from build123d import *

# Parameters (mm, degrees)
SKETCH2_R           = 14
BOSS_EXTRUDE1_DEPTH = 24
SKETCH3_R           = 3.95
BOSS_EXTRUDE2_DEPTH = 7
SKETCH4_R           = 3
BOSS_EXTRUDE3_DEPTH = 7
SKETCH6_R           = 1.25
CUT_EXTRUDE1_DEPTH  = 5
EXTRUDE_START       = 3
SKETCH_1_R          = 3
EXTRUDE_1_DEPTH     = 3
CUT_EXTRUDE2_START  = -5
CUT_EXTRUDE2_DEPTH  = 5


with BuildPart() as part:
    # Sketch2 → Boss-Extrude1 (new body)
    with BuildSketch(Plane(origin=(0, 0, 0), x_dir=(1, 0, 0), z_dir=(0, 1, 0))):
        with Locations(Location((0, 0, 0), (0, 0, 270))):
            Circle(SKETCH2_R)
    extrude(amount=BOSS_EXTRUDE1_DEPTH)

    # Sketch3 → Boss-Extrude2 (add)
    with BuildSketch(Plane(origin=(0, 24, 0), x_dir=(1, 0, 0), z_dir=(0, 1, 0))):
        with Locations(Location((0, 0, 0), (0, 0, 270))):
            Circle(SKETCH3_R)
    extrude(amount=BOSS_EXTRUDE2_DEPTH)

    # Sketch4 → Boss-Extrude3 (add)
    with BuildSketch(Plane(origin=(0, 31, 0), x_dir=(1, 0, 0), z_dir=(0, 1, 0))):
        with Locations(Location((0, 0, 0), (0, 0, 270))):
            Circle(SKETCH4_R)
    extrude(amount=BOSS_EXTRUDE3_DEPTH)

    # Sketch6 → Cut-Extrude1 (cut)
    with BuildSketch(Plane.XZ):
        with Locations(Location((8, 0, 0), (0, 0, 270))):
            Circle(SKETCH6_R)
        with Locations(Location((0, -8, 0), (0, 0, 270))):
            Circle(SKETCH6_R)
        with Locations(Location((-8, 0, 0), (0, 0, 270))):
            Circle(SKETCH6_R)
        with Locations(Location((0, 8, 0), (0, 0, 270))):
            Circle(SKETCH6_R)
    extrude(amount=-CUT_EXTRUDE1_DEPTH, mode=Mode.SUBTRACT)

    # 草图1 → 凸台-拉伸1 (add)
    with BuildSketch(Plane.XZ.offset(EXTRUDE_START)):
        with Locations(Location((0, 0, 0), (0, 0, 90))):
            Circle(SKETCH_1_R)
    extrude(amount=-EXTRUDE_1_DEPTH)

    # Sketch7 → Cut-Extrude2 (cut)
    with BuildSketch(Plane(origin=(0, 31, 0), x_dir=(1, 0, 0), z_dir=(0, 1, 0)).offset(CUT_EXTRUDE2_START)):
        with BuildLine():
            Line((-2.010596926, 3.4), (2.010596926, 3.4))
            ThreePointArc((2.010596926, 3.4), (0, 3.95), (-2.010596926, 3.4))
        make_face()
        with BuildLine():
            Line((-2.010596926, -3.4), (2.010596926, -3.4))
            ThreePointArc((2.010596926, -3.4), (0, -3.95), (-2.010596926, -3.4))
        make_face()
    extrude(amount=CUT_EXTRUDE2_DEPTH, mode=Mode.SUBTRACT)


solid = part.part
Part model, mm, in its own coordinate system. A direction names the side the tool comes from. Round coordinates to 2 decimals unless told otherwise and drop trailing zeros. Write each loop counter-clockwise with the first axis right and the second up, starting at its lowest first coordinate (ties: lowest second). Pieces come first, ordered by that corner, then holes. Notation, with made-up numbers: M -4.75,52.5 L 31.25,52.5 A24 cw 31.25,69.5 Z; hole C 1,-8 d2. An arc over 180 degrees is marked long. Return JSON: item names as keys, results as strings. Group by question number.
(1) Pin check, flat tips, straight feed: pin 1 Ø5 at (x, y) = (-7, 19.5) entering from -Z; pin 2 Ø8.5 at (x, z) = (5, 7) entering from +Y; pin 3 Ø3 at (x, z) = (0, 8) entering from -Y. Stop position of each tip, or through.
(2) Saw through at D-D on y = 18. Write the cut outline in (x, z), then the cut area to 3 significant figures.
(3) Which spindle directions (+Z, -Z, +X, -X, +Y, -Y) get a long thin tool onto all of the face, cutting with end or side? Do faces 1 (the face through (0.05, 2.46, 9.25)), 2 (the face through (0, 28, 3.4)), 3 (the face through (-3, 24, 3)). Say none if no direction does.
(4) Saw through at A-A on z = 0. Write the cut outline in (x, y), then the cut area to 3 significant figures.
(5) Two-plate mould, pull along Z, no slides. Class faces 4 (the face through (-9.22, 2.46, 0.27)), 5 (the face through (-3, 31, 1)), 6 (the face through (-13.67, 11.83, -3.03)): +Z half, -Z half, draft (parallel to the pull), parting line (faces both ways), or undercut.
(6) Saw through at C-C on x = 0. Write the cut outline in (y, z).
(7) Drill centre lines: probe 1 along X at (y, z) = (1.45, 0); probe 2 along Z at (x, y) = (1, 4); probe 3 along X at (y, z) = (3.1, -8). Where is each one in solid material? Low to high.
(8) Saw through at B-B on y = 4.5. Write the cut outline in (x, z), then the cut area to 3 significant figures.
Returned:
{
 "1": {"pin 1": "z = -13.26", "pin 2": "y = 24", "pin 3": "y = 0"},
 "2": {"outline": "C 0,0 d28", "area": "616 mm²"},
 "3": {"face 1": "-Y", "face 2": "+Z, +X, -X, +Y", "face 3": "+Y"},
 "4": {"outline": "M -14,0 L -9.25,0 L -9.25,5 L -6.75,5 L -6.75,0 L -3,0 L -3,-3 L 3,-3 L 3,0 L 6.75,0 L 6.75,5 L 9.25,5 L 9.25,0 L 14,0 L 14,24 L 3.95,24 L 3.95,31 L 3,31 L 3,38 L -3,38 L -3,31 L -3.95,31 L -3.95,24 L -14,24 Z", "area": "762 mm²"},
 "5": {"face 4": "undercut", "face 5": "draft", "face 6": "parting line"},
 "6": {"outline": "M -3,-3 L 0,-3 L 0,-6.75 L 5,-6.75 L 5,-9.25 L 0,-9.25 L 0,-14 L 24,-14 L 24,-3.95 L 26,-3.95 L 26,-3.4 L 31,-3.4 L 31,-3 L 38,-3 L 38,3 L 31,3 L 31,3.4 L 26,3.4 L 26,3.95 L 24,3.95 L 24,14 L 0,14 L 0,9.25 L 5,9.25 L 5,6.75 L 0,6.75 L 0,3 L -3,3 Z"},
 "7": {"probe 1": "-14 to -9.25, -6.75 to 6.75, 9.25 to 14", "probe 2": "-13.96 to -8.75, -7.25 to 7.25, 8.75 to 13.96", "probe 3": "-11.49 to -1.25, 1.25 to 11.49"},
 "8": {"outline": "C 0,0 d28; hole C -8,0 d2.5; hole C 0,-8 d2.5; hole C 0,8 d2.5; hole C 8,0 d2.5", "area": "596 mm²"}
}
